```python
from build123d import *

# Parameters (mm, degrees)
SKETCH_1_W             = 22
SKETCH_1_H             = 30
EXTRUDE_1_DEPTH        = 8
SKETCH_2_R             = 4.5
CUT_EXTRUDE_1_DEPTH    = 9
SKETCH_3_W             = 7
SKETCH_3_H             = 8
CUT_EXTRUDE_2_DEPTH    = 9
SKETCH_4_R             = 5.25
CUT_EXTRUDE_3_DEPTH    = 1
SKETCH_5_R             = 5.25
CUT_EXTRUDE_4_DEPTH    = 1
SKETCH_6_W             = 22
SKETCH_6_H             = 5
EXTRUDE_2_DEPTH        = 12
CUT_EXTRUDE_5_DEPTH    = 2.5
PATTERN_LINEAR_1_COUNT = 2
PATTERN_LINEAR_1_PITCH = 10
SKETCH_8_R             = 1.5
CUT_EXTRUDE_6_DEPTH    = 28.5
PATTERN_LINEAR_2_COUNT = 2
PATTERN_LINEAR_2_PITCH = 10


with BuildPart() as part:
    # 草图1 → 凸台-拉伸1 (new body)
    with BuildSketch(Plane(origin=(0, 0, 0), x_dir=(0, 0, -1), z_dir=(1, 0, 0))):
        Rectangle(SKETCH_1_W, SKETCH_1_H)
    extrude(amount=EXTRUDE_1_DEPTH)

    # 草图2 → 切除-拉伸1 (cut, through all)
    with BuildSketch(Plane.ZY):
        with Locations((0, 4)):
            Circle(SKETCH_2_R)
    extrude(amount=-CUT_EXTRUDE_1_DEPTH, mode=Mode.SUBTRACT)

    # 草图3 → 切除-拉伸2 (cut, through all)
    with BuildSketch(Plane.ZY):
        with Locations((7.5, -6)):
            Rectangle(SKETCH_3_W, SKETCH_3_H)
    extrude(amount=-CUT_EXTRUDE_2_DEPTH, mode=Mode.SUBTRACT)

    # 草图4 → 切除-拉伸3 (cut)
    with BuildSketch(Plane.ZY):
        with Locations((0, 4)):
            Circle(SKETCH_4_R)
    extrude(amount=-CUT_EXTRUDE_3_DEPTH, mode=Mode.SUBTRACT)

    # 草图5 → 切除-拉伸4 (cut)
    with BuildSketch(Plane(origin=(8, 0, 0), x_dir=(0, 0, -1), z_dir=(1, 0, 0))):
        with Locations((0, 4)):
            Circle(SKETCH_5_R)
    extrude(amount=-CUT_EXTRUDE_4_DEPTH, mode=Mode.SUBTRACT)

    # 草图6 → 凸台-拉伸2 (add)
    with BuildSketch(Plane(origin=(8, 0, 0), x_dir=(0, 0, -1), z_dir=(1, 0, 0))):
        with Locations((0, -12.5)):
            Rectangle(SKETCH_6_W, SKETCH_6_H)
    extrude(amount=EXTRUDE_2_DEPTH)

    # 草图7 → 切除-拉伸5 (cut)
    with BuildSketch(Plane.XZ.offset(15)):
        Polygon((9.8, -5), (11.4, -7.771281292), (14.6, -7.771281292), (16.2, -5), (14.6, -2.228718708), (11.4, -2.228718708), align=None)
    cut_extrude_5 = extrude(amount=-CUT_EXTRUDE_5_DEPTH, mode=Mode.SUBTRACT)

    # 阵列(线性)1: 切除-拉伸5 ×2
    with Locations(*[(0, 0, i * PATTERN_LINEAR_1_PITCH) for i in range(1, PATTERN_LINEAR_1_COUNT)]):
        add(cut_extrude_5, mode=Mode.SUBTRACT)

    # 草图8 → 切除-拉伸6 (cut, through all)
    with BuildSketch(Plane.XZ.offset(12.5)):
        with Locations((13, 5)):
            Circle(SKETCH_8_R)
    cut_extrude_6 = extrude(amount=-CUT_EXTRUDE_6_DEPTH, mode=Mode.SUBTRACT)

    # 阵列(线性)2: 切除-拉伸6 ×2
    with Locations(*[(0, 0, -i * PATTERN_LINEAR_2_PITCH) for i in range(1, PATTERN_LINEAR_2_COUNT)]):
        add(cut_extrude_6, mode=Mode.SUBTRACT)


solid = part.part
```
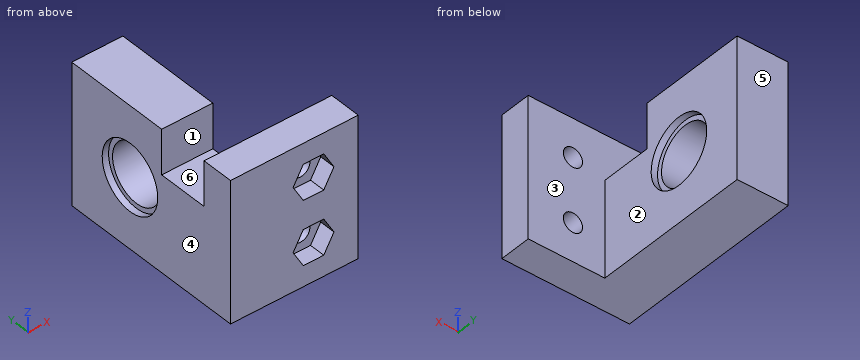
For this review, take the finished solid that the model builds, in its own axes (mm). Face numbers are marked on the shaded views. A direction names the side the tool comes from. Round coordinates to 2 decimals unless told otherwise and drop trailing zeros. Write each loop counter-clockwise with the first axis right and the second up, starting at its lowest first coordinate (ties: lowest second). Pieces come first, ordered by that corner, then holes. Notation, with made-up numbers: (-17.75, 40) - (-1.75, 40) arc R9 ccw to (-1.75, 54) - close; hole circle Ø6 at (-14, 26). An arc over 180 degrees is marked (long way). Answer as a JSON object with one key per item and string values.
1. We need section D-D on y = -11.5. Give the boundary of the cut face in (x, z).
Response values:
{"outline": "(0, -11) - (20, -11) - (20, 11) - (0, 11) - close; hole circle Ø3 at (13, -5); hole circle Ø3 at (13, 5)"}
2. We need section B-B on z = 9.75. Give the boundary of the cut face in (x, y).
Response values:
{"outline": "(0, -15) - (20, -15) - (20, -10) - (0, -10) - close; (0, -2) - (8, -2) - (8, 15) - (0, 15) - close"}
3. We need section A-A on x = 13. Give the boundary of the cut face in (y, z).
Response values:
{"outline": "(-15, -11) - (-10, -11) - (-10, -6.5) - (-12.5, -6.5) - (-12.5, -7.77) - (-15, -7.77) - close; (-15, -2.23) - (-12.5, -2.23) - (-12.5, -3.5) - (-10, -3.5) - (-10, 3.5) - (-12.5, 3.5) - (-12.5, 2.23) - (-15, 2.23) - close; (-15, 7.77) - (-12.5, 7.77) - (-12.5, 6.5) - (-10, 6.5) - (-10, 11) - (-15, 11) - close"}
4. Draft analysis for pull direction Y (two halves, no side actions). For the marked faces 4, 5 and 6, state which applies: +Y half, -Y half, draft (parallel to the pull), parting line (faces both ways), or undercut.
Response values:
{"face 4": "draft", "face 5": "+Y half", "face 6": "undercut"}
5. For pin 1 Ø9.5 at (y, z) = (4, 0) entering from -X; pin 2 Ø2 at (x, z) = (17, 8) entering from +Y; pin 3 Ø4 at (x, y) = (3, -4.5) entering from +Z; pin 4 Ø6 at (x, z) = (13.5, 5) entering from -Y, all flat-tipped, find the tip position at first contact; note any pin that passes through.
Response values:
{"pin 1": "stops at x = 1", "pin 2": "stops at y = -10", "pin 3": "stops at z = 4", "pin 4": "stops at y = -15"}
6. Tool access review of the marked faces 1, 2 and 3: name each direction out of +Z, -Z, +X, -X, +Y, -Y from which nothing blocks a thin tool from reaching the whole face with its end or side.
Response values:
{"face 1": "+Z, +X, -X", "face 2": "+Z, -Z, +X, +Y", "face 3": "+Z, +X"}
7. To check wall thickness, follow line 1 along Y through (x, z) = (3.25, 8.5); line 2 along Y through (x, z) = (5.8, 0); line 3 along X through (y, z) = (-4, -5.75). State the ranges of each line that lie inside material, in increasing order.
Response values:
{"line 1": "y = -15 to -10, -2 to 15", "line 2": "y = -15 to -0.5, 8.5 to 15", "line 3": "x = 0 to 8"}
8. We need section C-C on x = 1.75. Give the boundary of the cut face in (y, z), then the cut area to 3 significant figures.
Response values:
{"outline": "(-15, -11) - (15, -11) - (15, 11) - (-2, 11) - (-2, 4) - (-10, 4) - (-10, 11) - (-15, 11) - close; hole circle Ø9 at (4, 0)", "area": "540 mm2"}
